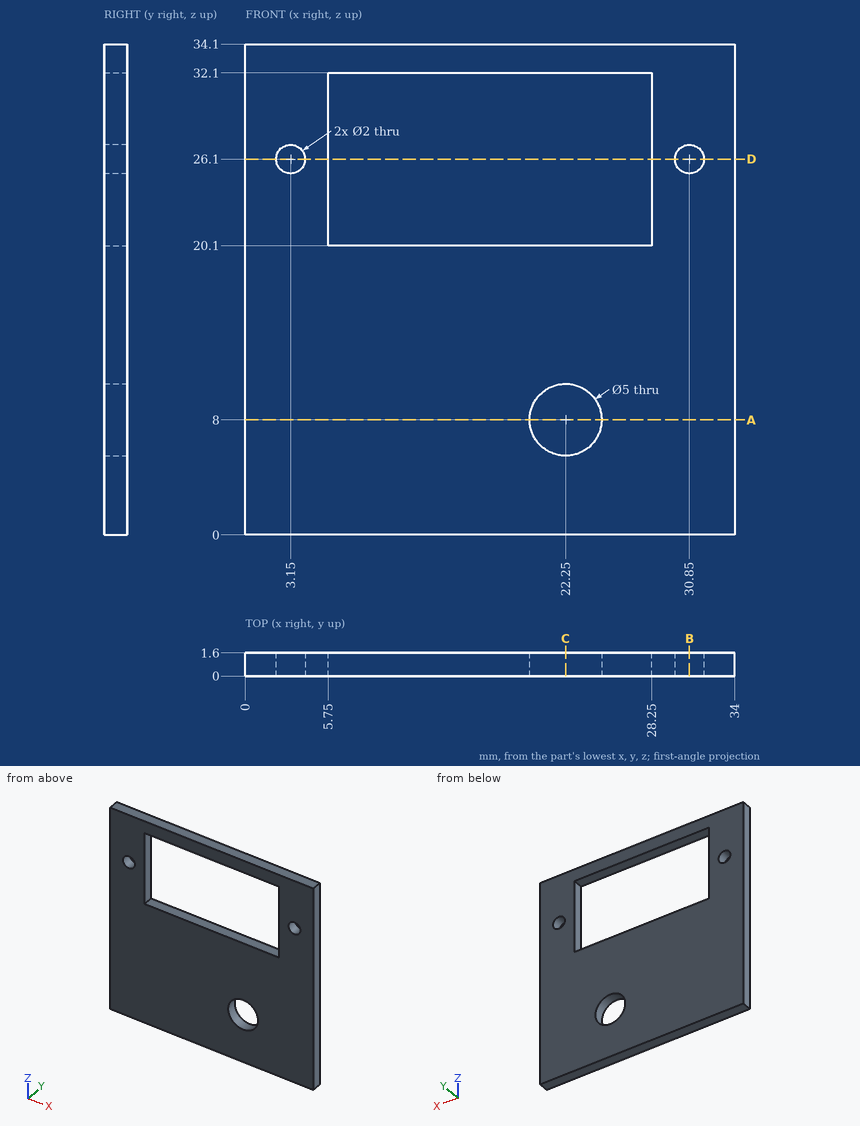
Job drawing, mm, ordinate dimensions from the low corner. One solid piece. Coordinates: 2 decimals unless noted, no trailing zeros. Order: outer loops, then holes, each group sorted by start corner. A loop starts at its lowest first (then second) coordinate and runs counter-clockwise, first axis right, second up. Notation, with made-up numbers: M 73.5,38 L 79.5,38 A23 cw 79.5,61 Z; hole C 4.25,77 d1. An arc over 180 degrees is marked long. Return JSON: item names as keys, results as strings.
1. Saw through at D-D (z = 26.1). Give the cut face in (x, y), and give its area (3 significant figures).
Ans:
{"outline": "M 0,0 L 2.15,0 L 2.15,1.6 L 0,1.6 Z; M 4.15,0 L 5.75,0 L 5.75,1.6 L 4.15,1.6 Z; M 28.25,0 L 29.85,0 L 29.85,1.6 L 28.25,1.6 Z; M 31.85,0 L 34,0 L 34,1.6 L 31.85,1.6 Z", "area": "12.0 mm^2"}
2. Saw through at C-C (x = 22.25). Give the cut face in (y, z).
Ans:
{"outline": "M 0,0 L 1.6,0 L 1.6,5.5 L 0,5.5 Z; M 0,10.5 L 1.6,10.5 L 1.6,20.1 L 0,20.1 Z; M 0,32.1 L 1.6,32.1 L 1.6,34.1 L 0,34.1 Z"}
3. Saw through at A-A (z = 8). Give the cut face in (x, y).
Ans:
{"outline": "M 0,0 L 19.75,0 L 19.75,1.6 L 0,1.6 Z; M 24.75,0 L 34,0 L 34,1.6 L 24.75,1.6 Z"}
4. Saw through at B-B (x = 30.85). Give the cut face in (y, z), and give its area (3 significant figures).
Ans:
{"outline": "M 0,0 L 1.6,0 L 1.6,25.1 L 0,25.1 Z; M 0,27.1 L 1.6,27.1 L 1.6,34.1 L 0,34.1 Z", "area": "51.4 mm^2"}
5. Flat gauge pin, fed straight in: pin 1 (3 mm diameter, centred on x = 22.25, z = 8, fed in from +Y). Where does the tip first touch, or does it go through?
Ans:
{"pin 1": "through"}
6. Drill centre lines: probe 1 along Z at (x, y) = (22.25, 0.4); probe 2 along Z at (x, y) = (18, 1.35); probe 3 along X at (y, z) = (0.7, 8). Where is each one in solid material? Low to high.
Ans:
{"probe 1": "0 to 5.5, 10.5 to 20.1, 32.1 to 34.1", "probe 2": "0 to 20.1, 32.1 to 34.1", "probe 3": "0 to 19.75, 24.75 to 34"}
